```python
from build123d import *

# Parameters (mm, degrees)
SKETCH_1_R      = 2
SKETCH_1_R_2    = 12
EXTRUDE_1_DEPTH = 1.5
FILLET_1_R      = 1


with BuildPart() as part:
    # ｽｹｯﾁ1 → ﾎﾞｽ - 押し出し1 (new body)
    with BuildSketch(Plane(origin=(0, 0, 0), x_dir=(1, 0, 0), z_dir=(0, 1, 0))):
        with BuildLine():
            Line((50, 24.75), (0, 24.75))
            ThreePointArc((0, 24.75), (-1.735055234, 24.197362526), (-2.830872774, 22.743055556))
            ThreePointArc((-2.830872774, 22.743055556), (-5.313420016, 18.286619233), (-9.145896655, 14.919871795))
            ThreePointArc((-9.145896655, 14.919871795), (-12.374368671, 12.374368671), (-14.919871795, 9.145896655))
            ThreePointArc((-14.919871795, 9.145896655), (-18.286619233, 5.313420016), (-22.743055556, 2.830872774))
            ThreePointArc((-22.743055556, 2.830872774), (-24.75, 0), (-22.743055556, -2.830872774))
            ThreePointArc((-22.743055556, -2.830872774), (-18.286619233, -5.313420016), (-14.919871795, -9.145896655))
            ThreePointArc((-14.919871795, -9.145896655), (-12.374368671, -12.374368671), (-9.145896655, -14.919871795))
            ThreePointArc((-9.145896655, -14.919871795), (-5.313420016, -18.286619233), (-2.830872774, -22.743055556))
            ThreePointArc((-2.830872774, -22.743055556), (0, -24.75), (2.830872774, -22.743055556))
            ThreePointArc((2.830872774, -22.743055556), (5.313420016, -18.286619233), (9.145896655, -14.919871795))
            ThreePointArc((9.145896655, -14.919871795), (15.269302398, -8.54976048), (17.5, 0))
            Line((17.5, 0), (32.5, 0))
            ThreePointArc((32.5, 0), (34.730697602, -8.54976048), (40.854103345, -14.919871795))
            ThreePointArc((40.854103345, -14.919871795), (44.686579984, -18.286619233), (47.169127226, -22.743055556))
            ThreePointArc((47.169127226, -22.743055556), (50, -24.75), (52.830872774, -22.743055556))
            ThreePointArc((52.830872774, -22.743055556), (55.313420016, -18.286619233), (59.145896655, -14.919871795))
            ThreePointArc((59.145896655, -14.919871795), (62.374368671, -12.374368671), (64.919871795, -9.145896655))
            ThreePointArc((64.919871795, -9.145896655), (68.286619233, -5.313420016), (72.743055556, -2.830872774))
            ThreePointArc((72.743055556, -2.830872774), (74.75, 0), (72.743055556, 2.830872774))
            ThreePointArc((72.743055556, 2.830872774), (68.286619233, 5.313420016), (64.919871795, 9.145896655))
            ThreePointArc((64.919871795, 9.145896655), (62.374368671, 12.374368671), (59.145896655, 14.919871795))
            ThreePointArc((59.145896655, 14.919871795), (55.313420016, 18.286619233), (52.830872774, 22.743055556))
            ThreePointArc((52.830872774, 22.743055556), (51.735055234, 24.197362526), (50, 24.75))
        make_face()
        with Locations(Location((0, 21.75, 0), (0, 0, 270))):
            Circle(SKETCH_1_R, mode=Mode.SUBTRACT)
        with Locations(Location((50, 21.75, 0), (0, 0, 270))):
            Circle(SKETCH_1_R, mode=Mode.SUBTRACT)
        with Locations(Location((0, 0, 0), (0, 0, 270))):
            Circle(SKETCH_1_R_2, mode=Mode.SUBTRACT)
        with Locations(Location((50, 0, 0), (0, 0, 270))):
            Circle(SKETCH_1_R_2, mode=Mode.SUBTRACT)
        with Locations(Location((-21.75, 0, 0), (0, 0, 270))):
            Circle(SKETCH_1_R, mode=Mode.SUBTRACT)
        with Locations(Location((71.75, 0, 0), (0, 0, 270))):
            Circle(SKETCH_1_R, mode=Mode.SUBTRACT)
        with Locations(Location((0, -21.75, 0), (0, 0, 270))):
            Circle(SKETCH_1_R, mode=Mode.SUBTRACT)
        with Locations(Location((50, -21.75, 0), (0, 0, 270))):
            Circle(SKETCH_1_R, mode=Mode.SUBTRACT)
    extrude(amount=EXTRUDE_1_DEPTH)

    # ﾌｨﾚｯﾄ1
    fillet_1_edges = [part.edges().sort_by_distance(p)[0] for p in [
        (32.5, 0.75, 0),
        (17.5, 0.75, 0),
    ]]
    fillet(fillet_1_edges, radius=FILLET_1_R)


solid = part.part
```
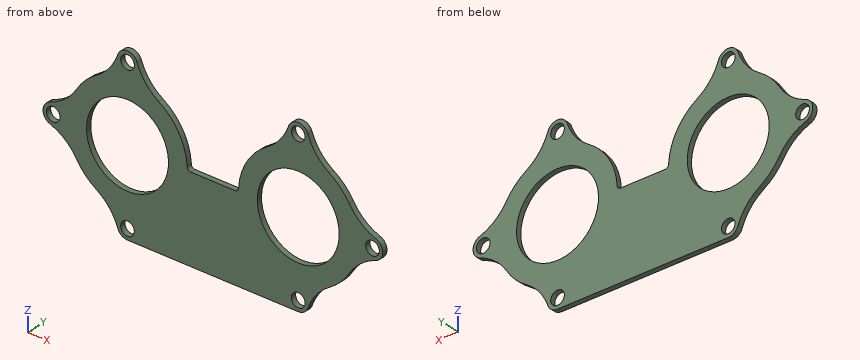
CAD build for the part. Positions are in the model's coordinates, mm. Give positions to 0.01 mm unless a question says otherwise; leave off trailing zeros. Write each loop counter-clockwise with the first axis right and the second up, starting at its lowest first coordinate (ties: lowest second). Pieces come first, ordered by that corner, then holes. Notation, with made-up numbers: (-11.75, 45.25) -> (-3.75, 45.25) arc R9 ccw to (-3.75, 54.25) -> close; hole circle Ø3 at (-27, 75). An arc over 180 degrees is marked (long way). Write each question's results on one line, items separated by ' | '.
1. Wall check: probe 1 along X at (y, z) = (0.7, -21.75); probe 2 along X at (y, z) = (1.1, -1); probe 3 along Z at (x, y) = (46.5, 0.5). Give the ranges that are in metal, low to high. Write a range as [from, to].
Geometry check:
probe 1: [-3.22, -2], [2, 48], [52, 53.22] | probe 2: [-24.58, -23.48], [-20.02, -11.96], [11.96, 38.04], [61.96, 70.02], [73.48, 74.58] | probe 3: [-24.75, -11.48], [11.48, 21.14]
2. Cut at A-A, the plane y = 0.55. Give the number of separate pieces and of enclosed holes in the cut face, then the cut area to 3 significant figures.
Geometry check:
separate pieces: 1 | enclosed holes: 8 | area: 1,990 mm²
3. Cut at B-B, the plane x = 51. Write the cut outline in (y, z), then the cut area to 3 significant figures.
Geometry check:
outline: (0, -24.58) -> (1.5, -24.58) -> (1.5, -23.48) -> (0, -23.48) -> close; (0, -20.02) -> (1.5, -20.02) -> (1.5, -11.96) -> (0, -11.96) -> close; (0, 11.96) -> (1.5, 11.96) -> (1.5, 20.02) -> (0, 20.02) -> close; (0, 23.48) -> (1.5, 23.48) -> (1.5, 24.58) -> (0, 24.58) -> close | area: 27.5 mm²
4. Cut at C-C, the plane z = 21.75. Write the cut outline in (x, y).
Geometry check:
outline: (-3.22, 0) -> (-2, 0) -> (-2, 1.5) -> (-3.22, 1.5) -> close; (2, 0) -> (3.22, 0) -> (3.22, 1.5) -> (2, 1.5) -> close; (46.78, 0) -> (48, 0) -> (48, 1.5) -> (46.78, 1.5) -> close; (52, 0) -> (53.22, 0) -> (53.22, 1.5) -> (52, 1.5) -> close
5. Drop a flat-ended pin along its axis: P1, Ø3, axis at x = 71.75, z = 0, coming from the +Y side. Give the stop position or say it passes through.
Geometry check:
P1: through
6. Cut at D-D, the plane x = -21.75. Write the cut outline in (y, z).
Geometry check:
outline: (0, -3.22) -> (1.5, -3.22) -> (1.5, -2) -> (0, -2) -> close; (0, 2) -> (1.5, 2) -> (1.5, 3.22) -> (0, 3.22) -> close
